The drawing under review shows one solid part. Ordinate dimensions are in mm from its lowest x, y, z. A direction names the side the tool comes from. Coordinates: 2 decimals unless noted, no trailing zeros. Write each loop counter-clockwise with the first axis right and the second up, starting at its lowest first coordinate (ties: lowest second). Pieces come first, ordered by that corner, then holes. Notation, with made-up numbers: M 60.25,19.5 L 96.25,19.5 A27 ccw 96.25,58.5 Z; hole C -17.5,-38 d4. An arc over 180 degrees is marked long. Write item = value, one per line.
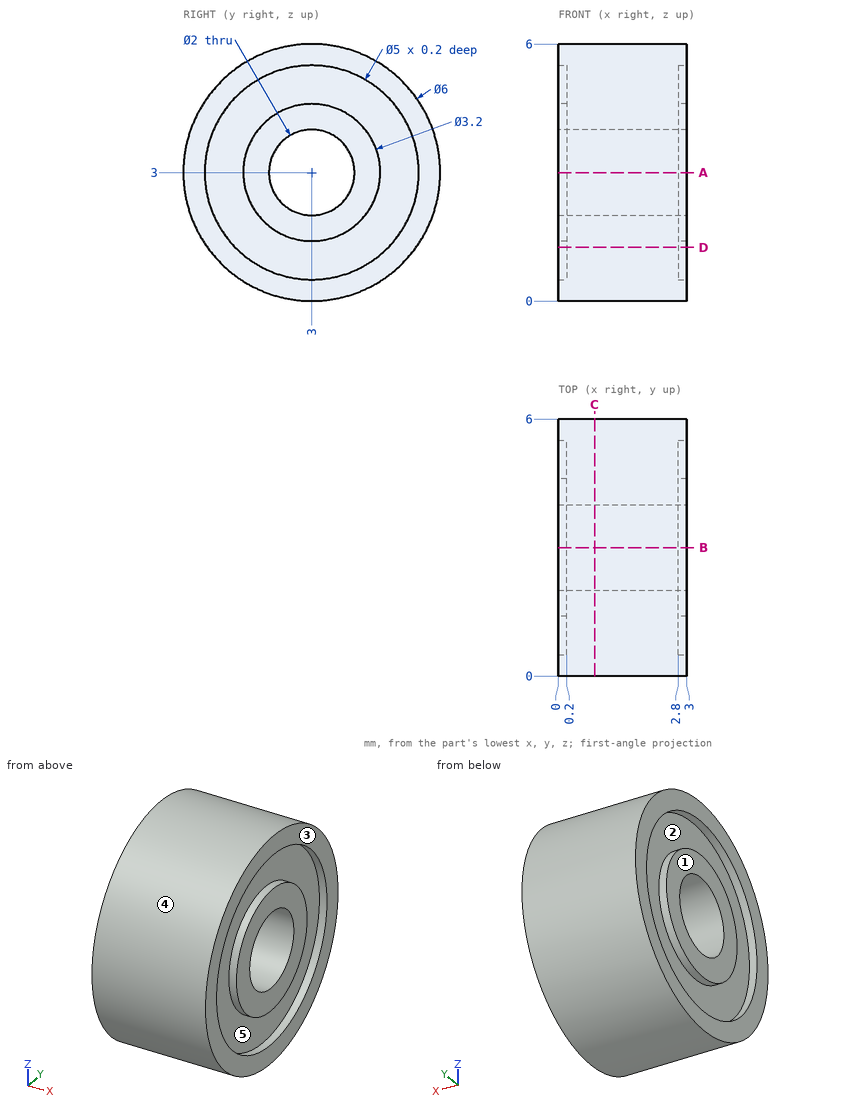
Q1. The part is to be moulded in two halves that separate along Z. For the marked faces 3, 4 and 5, say which applies: +Z half, -Z half, draft (parallel to the pull), parting line (faces both ways), or undercut.
Check result:
face_3 = draft
face_4 = parting line
face_5 = undercut
Q2. Consider section C-C, the plane x = 0.85. State the section outline as (y, z) points, and give its area (3 significant figures).
Check result:
outline = C 3,3 d6; hole C 3,3 d2
area = 25.1 mm²
Q3. Consider section D-D, the plane z = 1.25. State the section outline as (x, y) points.
Check result:
outline = M 0,0.56 L 3,0.56 L 3,1.21 L 2.8,1.21 L 2.8,4.79 L 3,4.79 L 3,5.44 L 0,5.44 L 0,4.79 L 0.2,4.79 L 0.2,1.21 L 0,1.21 Z
Q4. Consider section A-A, the plane z = 3. State the section outline as (x, y) points, and give its area (3 significant figures).
Check result:
outline = M 0,0 L 3,0 L 3,0.5 L 2.8,0.5 L 2.8,1.4 L 3,1.4 L 3,2 L 0,2 L 0,1.4 L 0.2,1.4 L 0.2,0.5 L 0,0.5 Z; M 0,4 L 3,4 L 3,4.6 L 2.8,4.6 L 2.8,5.5 L 3,5.5 L 3,6 L 0,6 L 0,5.5 L 0.2,5.5 L 0.2,4.6 L 0,4.6 Z
area = 11.3 mm²
Q5. Machinability: for the marked faces 1 and 2, which of the approach directions +Z, -Z, +X, -X, +Y, -Y give a long, thin tool a straight path to every point of the face, cutting with its end or side? Answer none if there is none.
Check result:
face_1 = +Z, -Z, -X, +Y, -Y
face_2 = -X
Q6. For P1, Ø1, axis at x = 1, y = 1.5, coming from the +Z side, flat-tipped, find the tip position at first contact; note if it passes through.
Check result:
P1 = 5.83
Q7. Wall thickness on line 1 (Y direction, x = 2.95, z = 3); line 2 (Y direction, x = 1.1, z = 3): over which ranges is each line inside the solid? List them lowest first.
Check result:
line_1 = 0 to 0.5, 1.4 to 2, 4 to 4.6, 5.5 to 6
line_2 = 0 to 2, 4 to 6
